Here's how the part is built. I have some questions about the finished solid (model axes, mm). Coordinates: 2 decimals unless noted, no trailing zeros. Write each loop counter-clockwise with the first axis right and the second up, starting at its lowest first coordinate (ties: lowest second). Pieces come first, ordered by that corner, then holes.
Item 1: I'm going to push flat-ended pins straight in: P1, Ø5.5, axis at x = -88.5, z = -163, coming from the -Y side; P2, Ø11, axis at x = -88.5, z = -159.5, coming from the +Y side; P3, Ø3, axis at x = -90, y = 268, coming from the -Z side; P4, Ø8, axis at x = -97, y = 279, coming from the -Z side. Where does each tip first touch, or does it pass through?
Item 2: I want a section at C-C (y = 289.5). Please give me the cut outline in (x, z).
Item 3: Please list where these lines run through material, in increasing order: line 1 (Z direction, x = -100.75, y = 290); line 2 (Y direction, x = -91, z = -111); line 3 (X direction, y = 283.5, z = -170).
Item 4: I want a section at B-B (x = -88.75). Please give me the cut outline in (y, z), and give its area (3 significant figures).
Item 5: I want a section at A-A (z = -123). Please give me the cut outline in (x, y).
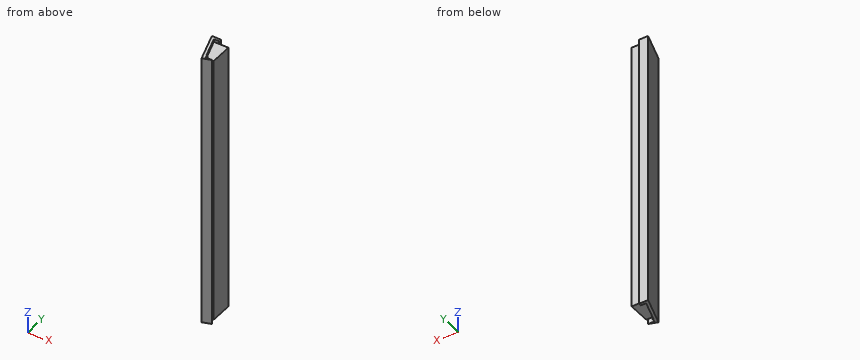
from build123d import *

# Parameters (mm, degrees)
BOSS_EXTRUDE1_DEPTH = 300
CUT_EXTRUDE1_DEPTH  = 3
CUT_EXTRUDE2_DEPTH  = 3


with BuildPart() as part:
    # Sketch1 → Boss-Extrude1 (new body)
    with BuildSketch(Plane.XY):
        Polygon((-105.938079236, 296), (-95.173448736, 262.988466467), (-85.938079236, 266), (-93, 266), (-93, 269), (-85.938079236, 269), (-85.938079236, 293), (-95.938079236, 293), (-95.938079236, 296), align=None)
    extrude(amount=-BOSS_EXTRUDE1_DEPTH)

    # Sketch2 → Cut-Extrude1 (cut)
    with BuildSketch(Plane(origin=(0, 0, -300), x_dir=(-1, 0, 0), z_dir=(0, 0, -1))):
        Polygon((93, 269), (93.97826087, 269), (101.804347826, 293), (95.938079236, 293), (85.938079236, 293), (85.938079236, 269), align=None)
    extrude(amount=-CUT_EXTRUDE1_DEPTH, mode=Mode.SUBTRACT)

    # Sketch3 → Cut-Extrude2 (cut)
    with BuildSketch(Plane.XY):
        Polygon((-101.804347826, 293), (-93.97826087, 269), (-93, 269), (-85.938079236, 269), (-85.938079236, 293), (-95.938079236, 293), align=None)
    extrude(amount=-CUT_EXTRUDE2_DEPTH, mode=Mode.SUBTRACT)


solid = part.part
Answer:
1. P1: stops at y = 264.27
1. P2: stops at y = 293
1. P3: stops at z = -297
1. P4: stops at z = -300
2. outline: (-103.82, -300) - (-100.66, -300) - (-100.66, -297) - (-85.94, -297) - (-85.94, -3) - (-100.66, -3) - (-100.66, 0) - (-103.82, 0) - close
3. line 1: z = -297 to -3
3. line 2: y = 264.35 to 266, 269 to 293
3. line 3: x = -101.86 to -85.94
4. outline: (265.08, -300) - (266, -300) - (266, 0) - (265.08, 0) - close; (269, -297) - (293, -297) - (293, -3) - (269, -3) - close
4. area: 7,330 mm2
5. outline: (-105.94, 296) - (-95.17, 262.99) - (-85.94, 266) - (-93, 266) - (-93, 269) - (-85.94, 269) - (-85.94, 293) - (-95.94, 293) - (-95.94, 296) - close
